The model under review builds one solid part; all positions refer to its coordinate system, in mm. A direction names the side the tool comes from. Round coordinates to 2 decimals unless told otherwise and drop trailing zeros. Loops run counter-clockwise (first coordinate to the right, second up) from the corner with the lowest first, then second, coordinate; pieces in that order, holes last. Notation, with made-up numbers: M 36,43 L 85,43 A11 ccw 85,61 Z; hole C 66.5,87.5 d7. An arc over 180 degrees is marked long. One line per question, with ' | ' between items.
from build123d import *

# Parameters (mm, degrees)
SKETCH1_R                 = 25
BOSS_EXTRUDE1_DEPTH       = 6
CUT_EXTRUDE1_REACH        = 37.861
SKETCH2_R                 = 10.5
SKETCH3_R                 = 2.5
CUT_EXTRUDE2_DEPTH        = 36.860842154
SKETCH5_R                 = 1.25
CUT_EXTRUDE3_DEPTH        = 4
BOSS_EXTRUDE2_START       = 1.5
SKETCH6_R                 = 26.576681464
SKETCH6_R_2               = 10.5
SKETCH6_R_3               = 1.25
BOSS_EXTRUDE2_DEPTH       = 1.5
SKETCH7_R                 = 4.5
CUT_EXTRUDE4_DEPTH        = 5
SKETCH8_R                 = 2.5
BOSS_EXTRUDE3_DEPTH       = 3
M3X0_5_TAPPED_HOLE1_D     = 2.5
M3X0_5_TAPPED_HOLE1_DEPTH = 5
M3X0_5_TAPPED_HOLE1_TIP   = 0.751075774


with BuildPart() as part:
    # Sketch1 → Boss-Extrude1 (new body)
    with BuildSketch(Plane(origin=(0, 0, 0), x_dir=(1, 0, 0), z_dir=(0, 1, 0))):
        with Locations(Location((0, 0, 0), (0, 0, 270))):
            Circle(SKETCH1_R)
    extrude(amount=BOSS_EXTRUDE1_DEPTH)

    # Sketch2 → Cut-Extrude1 (cut, up to next)
    with BuildSketch(Plane(origin=(0, 6, 0), x_dir=(1, 0, 0), z_dir=(0, 1, 0)), mode=Mode.PRIVATE) as cut_extrude1_sk1:
        with Locations(Location((0, 0, 0), (0, 0, 270))):
            Circle(SKETCH2_R)
    cut_extrude1_tool1 = extrude(cut_extrude1_sk1.sketch, amount=-CUT_EXTRUDE1_REACH, mode=Mode.PRIVATE) & part.part
    add(cut_extrude1_tool1.solids().sort_by_distance((0, 6, 0))[0], mode=Mode.SUBTRACT)

    # Sketch3 → Cut-Extrude2 (cut, through all)
    with BuildSketch(Plane(origin=(0, 6, 0), x_dir=(1, 0, 0), z_dir=(0, 1, 0))):
        with Locations(Location((0, 19, 0), (0, 0, 270))):
            Circle(SKETCH3_R)
        with Locations(Location((16.454482672, 9.5, 0), (0, 0, 270))):
            Circle(SKETCH3_R)
        with Locations(Location((16.454482672, -9.5, 0), (0, 0, 270))):
            Circle(SKETCH3_R)
        with Locations(Location((0, -19, 0), (0, 0, 270))):
            Circle(SKETCH3_R)
        with Locations(Location((-16.454482672, -9.5, 0), (0, 0, 270))):
            Circle(SKETCH3_R)
        with Locations(Location((-16.454482672, 9.5, 0), (0, 0, 270))):
            Circle(SKETCH3_R)
    extrude(amount=-CUT_EXTRUDE2_DEPTH, mode=Mode.SUBTRACT)

    # Sketch5 → Cut-Extrude3 (cut)
    with BuildSketch(Plane(origin=(0, 6, 0), x_dir=(1, 0, 0), z_dir=(0, 1, 0))):
        with Locations(Location((20, 0, 0), (0, 0, 270))):
            Circle(SKETCH5_R)
        with Locations(Location((10, -17.320508076, 0), (0, 0, 270))):
            Circle(SKETCH5_R)
        with Locations(Location((-10, -17.320508076, 0), (0, 0, 270))):
            Circle(SKETCH5_R)
        with Locations(Location((-20, 0, 0), (0, 0, 270))):
            Circle(SKETCH5_R)
        with Locations(Location((-10, 17.320508076, 0), (0, 0, 270))):
            Circle(SKETCH5_R)
        with Locations(Location((10, 17.320508076, 0), (0, 0, 270))):
            Circle(SKETCH5_R)
    extrude(amount=-CUT_EXTRUDE3_DEPTH, mode=Mode.SUBTRACT)

    # Sketch6 → Boss-Extrude2 (add)
    with BuildSketch(Plane(origin=(0, 6, 0), x_dir=(1, 0, 0), z_dir=(0, 1, 0)).offset(BOSS_EXTRUDE2_START)):
        with Locations(Location((0, 0, 0), (0, 0, 270))):
            Circle(SKETCH6_R)
        with Locations(Location((0, 0, 0), (0, 0, 270))):
            Circle(SKETCH6_R_2, mode=Mode.SUBTRACT)
        with Locations(Location((10, -17.320508076, 0), (0, 0, 270))):
            Circle(SKETCH6_R_3, mode=Mode.SUBTRACT)
        with Locations(Location((-10, -17.320508076, 0), (0, 0, 270))):
            Circle(SKETCH6_R_3, mode=Mode.SUBTRACT)
        with Locations(Location((-20, 0, 0), (0, 0, 270))):
            Circle(SKETCH6_R_3, mode=Mode.SUBTRACT)
        with Locations(Location((-10, 17.320508076, 0), (0, 0, 270))):
            Circle(SKETCH6_R_3, mode=Mode.SUBTRACT)
        with Locations(Location((10, 17.320508076, 0), (0, 0, 270))):
            Circle(SKETCH6_R_3, mode=Mode.SUBTRACT)
        with Locations(Location((20, 0, 0), (0, 0, 270))):
            Circle(SKETCH6_R_3, mode=Mode.SUBTRACT)
    extrude(amount=-BOSS_EXTRUDE2_DEPTH)

    # Sketch7 → Cut-Extrude4 (cut)
    with BuildSketch(Plane(origin=(0, 7.5, 0), x_dir=(1, 0, 0), z_dir=(0, 1, 0))):
        with Locations(Location((16.454482672, -9.5, 0), (0, 0, 270))):
            Circle(SKETCH7_R)
        with Locations(Location((-16.454482672, -9.5, 0), (0, 0, 270))):
            Circle(SKETCH7_R)
        with Locations(Location((0, 19, 0), (0, 0, 270))):
            Circle(SKETCH7_R)
    extrude(amount=-CUT_EXTRUDE4_DEPTH, mode=Mode.SUBTRACT)

    # Sketch8 → Boss-Extrude3 (add)
    with BuildSketch(Plane.XZ.offset(-6)):
        with Locations(Location((0, 19, 0), (0, 0, 90))):
            Circle(SKETCH8_R)
        with Locations(Location((16.454482672, -9.5, 0), (0, 0, 90))):
            Circle(SKETCH8_R)
        with Locations(Location((-16.454482672, -9.5, 0), (0, 0, 90))):
            Circle(SKETCH8_R)
    extrude(amount=BOSS_EXTRUDE3_DEPTH)

    # M3x0.5 Tapped Hole1
    with Locations(Plane(origin=(0, 7.5, 0), x_dir=(1, 0, 0), z_dir=(0, 1, 0))):
        with Locations((-10, 17.320508076), (-20, 0), (-10, -17.320508076), (10, 17.320508076), (20, 0), (10, -17.320508076)):
            Hole(M3X0_5_TAPPED_HOLE1_D / 2, depth=M3X0_5_TAPPED_HOLE1_DEPTH)
            with Locations((0, 0, -(M3X0_5_TAPPED_HOLE1_DEPTH + M3X0_5_TAPPED_HOLE1_TIP / 2))):  # 118° drill point
                Cone(0, M3X0_5_TAPPED_HOLE1_D / 2, M3X0_5_TAPPED_HOLE1_TIP, mode=Mode.SUBTRACT)


solid = part.part
1) For line 1 (Z direction, x = -3.5, y = 4); line 2 (X direction, y = 3.25, z = 8); line 3 (Z direction, x = 20, y = 6.5), list the stretches that pass through material, from the lowest coordinate up.
Output values:
line 1: z = -24.75 to -21.83, -16.17 to -9.9, 9.9 to 24.75 | line 2: x = -23.69 to -20.7, -12.21 to -6.8, 6.8 to 12.21, 20.7 to 23.69 | line 3: z = -17.5 to -1.25, 1.25 to 6.73, 12.27 to 17.5
2) Add section C-C on y = 0.75. State the section outline as (x, z) points.
Output values:
outline: C 0,0 d50; hole C -16.45,-9.5 d5; hole C -16.45,9.5 d5; hole C 0,0 d21; hole C 0,-19 d5; hole C 0,19 d5; hole C 16.45,-9.5 d5; hole C 16.45,9.5 d5
3) Insertion check: P1, Ø3, axis at y = 4, z = 2, coming from the +X side (3 decimals); P2, Ø3, axis at x = 12.5, y = 5.5, coming from the -Z side; P3, Ø1.5, axis at y = 5, z = 17.5, coming from the +X side. Each pin has a flat end and moves straight along its axis. Give the tip position at first contact, or say it passes through.
Output values:
P1: stops at x = 24.995 | P2: stops at z = -24.15 | P3: stops at x = 18.56
4) Add section D-D on y = 3.75. State how many separate pieces and enclosed holes the cut face has, then the cut area to 3 significant figures.
Output values:
separate pieces: 1 | enclosed holes: 10 | area: 1,400 mm²
5) Add section A-A on x = 0. State the section outline as (y, z) points.
Output values:
outline: M 0,-25 L 6,-25 L 6,-26.58 L 7.5,-26.58 L 7.5,-23.5 L 2.5,-23.5 L 2.5,-21.5 L 0,-21.5 Z; M 0,-16.5 L 2.5,-16.5 L 2.5,-14.5 L 7.5,-14.5 L 7.5,-10.5 L 0,-10.5 Z; M 0,10.5 L 7.5,10.5 L 7.5,26.58 L 6,26.58 L 6,25 L 0,25 L 0,21.5 L 3,21.5 L 3,16.5 L 0,16.5 Z
6) Add section B-B on z = 6. State the section outline as (x, y) points.
Output values:
outline: M -25.89,6 L -24.27,6 L -24.27,0 L -8.62,0 L -8.62,7.5 L -13.63,7.5 L -13.63,2.5 L -19.28,2.5 L -19.28,7.5 L -25.89,7.5 Z; M 8.62,0 L 24.27,0 L 24.27,6 L 25.89,6 L 25.89,7.5 L 19.28,7.5 L 19.28,2.5 L 13.63,2.5 L 13.63,7.5 L 8.62,7.5 Z
7) Machinability: for faces 1 (the cylindrical face through (0.1, 1.3, -21.5)), 2 (the cylindrical face through (7.509, 2.958, 23.846)), 3 (the cylindrical face through (-12.66, 5.04, 11.92)), which of the approach directions +Z, -Z, +X, -X, +Y, -Y give a long, thin tool a straight path to every point of the face, cutting with its end or side? Answer none if there is none.
Output values:
face 1: +Y, -Y | face 2: -Y | face 3: +Y
8) Mouldability with a two-part tool opening along X and no side actions: class faces 4 (the flat face through (-11, 7.5, 0)), 5 (the cylindrical face through (-25.945, 6.76, -5.761)), 6 (the cylindrical face through (12.462, 5.035, 11.576)), 7 (the flat face through (14.5, 2.5, 11.4)) as +X half, -X half, draft (parallel to the pull), parting line (faces both ways), or undercut.
Output values:
face 4: draft | face 5: parting line | face 6: undercut | face 7: undercut
